```python
from build123d import *

# Parameters (mm, degrees)
F2_R     = 5
F3_DEPTH = 500
F4_R     = 5
F5_DEPTH = 5
F6_R     = 5
F7_DEPTH = 5


with BuildPart() as f1:
    # F0 (on Front) → F1 (revolve)
    with BuildSketch(Plane.XZ):
        Polygon((-0.16488, 15.599042), (-0.16488, 58.469787), (-49.661098, 58.469787), (-49.661098, 50.285377), (-42.645885, 44.439362), (-42.645885, 15.599042), (-42.645885, -13.241278), (-49.661098, -19.087292), (-49.661098, -27.271703), (-0.16488, -27.271703), align=None)
    revolve(axis=Axis((-0.16488, 0, 15.599042), (0, 0, -1)))

    # F2 (on Top) → F3 (cut, symmetric)
    with BuildSketch(Plane.XY):
        Circle(F2_R)
    extrude(amount=F3_DEPTH, both=True, mode=Mode.SUBTRACT)

    # F4 (on face) → F5 (cut)
    with BuildSketch(Plane.XY.offset(58.469787)):
        Circle(F4_R)
        Polygon((-4.34874, 9.196665), (-10.221355, 0.975004), (-6.037496, -8.221661), (4.01898, -9.196665), (9.891596, -0.975004), (5.707736, 8.221661), align=None)
        Circle(F4_R, mode=Mode.SUBTRACT)
    extrude(amount=-F5_DEPTH, mode=Mode.SUBTRACT)

    # F6 (on face) → F7 (cut)
    with BuildSketch(Plane(origin=(0, 0, -27.271703), x_dir=(1, 0, 0), z_dir=(0, 0, -1))):
        Polygon((2.242914, -9.851531), (9.653134, -2.983345), (7.410219, 6.868186), (-2.242914, 9.851531), (-9.653134, 2.983345), (-7.410219, -6.868186), align=None)
        Circle(F6_R, mode=Mode.SUBTRACT)
    extrude(amount=-F7_DEPTH, mode=Mode.SUBTRACT)


solid = f1.part
```
The model under review builds one solid part; all positions refer to its coordinate system, in mm. A direction names the side the tool comes from. Give positions to 0.01 mm unless a question says otherwise; leave off trailing zeros. Write each loop counter-clockwise with the first axis right and the second up, starting at its lowest first coordinate (ties: lowest second). Pieces come first, ordered by that corner, then holes.
(1) Consider section B-B, the plane z = 46. Give the boundary of the cut face in (x, y), and give its area (3 significant figures).
(2) Consider section A-A, the plane z = 11. Give the boundary of the cut face in (x, y).
(3) The part is to be moulded in two halves that separate along X. For faces 1 (the cylindrical face through (-47.375, 14.867, -23.237)), 2 (the flat face through (10, 1, 58.47)), 3 (the flat face through (-2, -5, -22.272)), say which applies: released by +X, released by -X, zero draft, split by the parting line, or undercut.
(4) For P1, Ø12, axis at x = 39.5, y = 34, coming from the +Z side; P2, Ø12, axis at x = -15.5, z = -5.5, coming from the +Y side; P3, Ø8, axis at y = -10.5, z = 20, coming from the -X side; P4, Ø6, axis at x = 11, z = 10.5, coming from the -Y side, all flat-tipped, find the tip position at first contact; note any pin that passes through.
(5) Tool access review of faces 4 (the cylindrical face through (-1.08, -4.88, 16.13)), 5 (the flat face through (6.914, -5.143, 56.005)), 6 (the flat face through (5.896, 6.466, -24.807)), 7 (the conical face through (5.422, 42.555, -13.607)): name each direction out of +Z, -Z, +X, -X, +Y, -Y from which nothing blocks a thin tool from reaching the whole face with its end or side.
(6) To check wall thickness, follow L1, parallel to Y at x = 0, z = 19; L2, parallel to Z at x = 17, y = -42.5; L3, parallel to Z at x = -36, y = -24. State the ranges of each line that lie inside material, in increasing order.
Returned:
1. outline: circle Ø88.71 at (-0.16, 0); hole circle Ø10 at (0, 0)
1. area: 6,100 mm2
2. outline: circle Ø84.96 at (-0.16, 0); hole circle Ø10 at (0, 0)
3. face 1: split by the parting line
3. face 2: zero draft
3. face 3: undercut
4. P1: stops at z = 58.47
4. P2: stops at y = 41.44
4. P3: stops at x = -42.15
4. P4: stops at y = -41.69
5. face 4: +Z, -Z
5. face 5: +Z
5. face 6: -Z
5. face 7: none
6. L1: y = -42.48 to -5, 5 to 42.48
6. L2: z = -27.27 to -16.04, 47.23 to 58.47
6. L3: z = -27.27 to -13.78, 44.98 to 58.47
